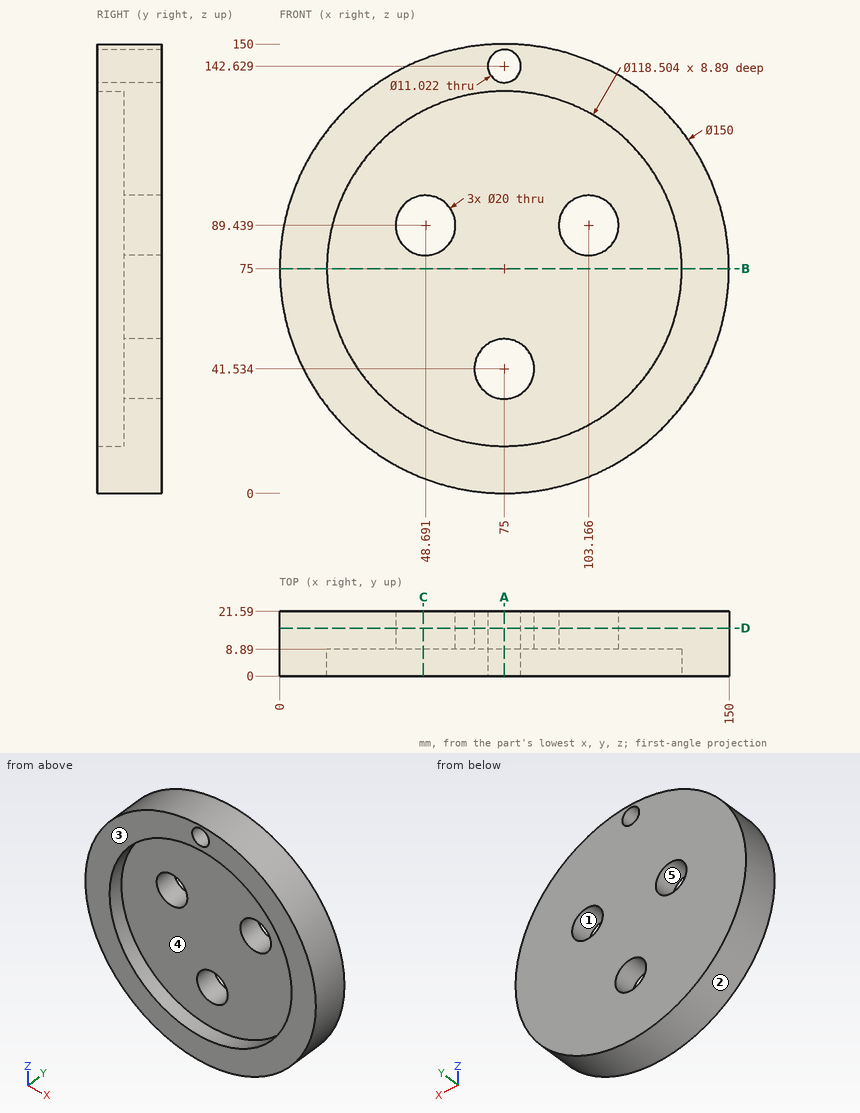
Can you work these out from the drawing? Everything is in mm from the part's minimum corner. A direction names the side the tool comes from. Round coordinates to 2 decimals unless told otherwise and drop trailing zeros. Write each loop counter-clockwise with the first axis right and the second up, starting at its lowest first coordinate (ties: lowest second). Pieces come first, ordered by that corner, then holes. Notation, with made-up numbers: (8.5, 45.5) - (63.5, 45.5) arc R20 cw to (63.5, 74.5) - close; hole circle Ø2 at (23.5, 62.25). An arc over 180 degrees is marked (long way). Put each result on its own line as item: value. Start each with the question number.
(1) Thinking about a two-plate mould opening in X: for the marked faces 1, 2 and 3, which applies, released by +X, released by -X, zero draft, split by the parting line, or undercut?
(2) I want a section at A-A, the plane x = 75. Please give me the cut outline in (y, z), plus the area to 3 significant figures.
(3) For the marked faces 4 and 5, which set-ups out of +Z, -Z, +X, -X, +Y, -Y let a thin tool reach every point of the face, with its end or its side?
(4) Will these pins go through, and if not, where does the flat tip stop? pin 1 (1 mm diameter, centred on x = 59, y = 17.5, fed in from +Z); pin 2 (1 mm diameter, centred on y = 18, z = 98.5, fed in from -X); pin 3 (3 mm diameter, centred on x = 57, z = 67.5, fed in from -Y); pin 4 (23 mm diameter, centred on x = 48.69, z = 89.44, fed in from +Y).
(5) I want a section at C-C, the plane x = 48. Please give me the cut outline in (y, z) (1 decimal).
(6) I need wall thicknesses on probe 1 along Z at (x, y) = (75, 2.5); probe 2 along Z at (x, y) = (77, 20.5) (1 decimal); probe 3 along Y at (x, z) = (102, 57). Which ranges of each line are inside material? Lowest first, please.
(7) I want a section at B-B, the plane z = 75. Please give me the cut outline in (x, y), plus the area to 4 significant figures.
(8) I want a section at D-D, the plane y = 16. Please give me the cut outline in (x, z).
Here are the results:
1. face 1: undercut
1. face 2: split by the parting line
1. face 3: zero draft
2. outline: (0, 0) - (21.59, 0) - (21.59, 31.53) - (8.89, 31.53) - (8.89, 15.75) - (0, 15.75) - close; (0, 134.25) - (8.89, 134.25) - (8.89, 51.53) - (21.59, 51.53) - (21.59, 137.12) - (0, 137.12) - close; (0, 148.14) - (21.59, 148.14) - (21.59, 150) - (0, 150) - close
2. area: 1,690 mm^2
3. face 4: -Y
3. face 5: +Y, -Y
4. pin 1: stops at z = 148.38
4. pin 2: stops at x = 3.61
4. pin 3: stops at y = 8.89
4. pin 4: stops at y = 21.59
5. outline: (0, 5) - (21.6, 5) - (21.6, 79.5) - (8.9, 79.5) - (8.9, 22.3) - (0, 22.3) - close; (0, 127.7) - (8.9, 127.7) - (8.9, 99.4) - (21.6, 99.4) - (21.6, 145) - (0, 145) - close
6. probe 1: z = 0 to 15.75, 134.25 to 137.12, 148.14 to 150
6. probe 2: z = 0 to 31.7, 51.3 to 137.5, 147.8 to 150
6. probe 3: y = 8.89 to 21.59
7. outline: (0, 0) - (15.75, 0) - (15.75, 8.89) - (134.25, 8.89) - (134.25, 0) - (150, 0) - (150, 21.59) - (0, 21.59) - close
7. area: 2,185 mm^2
8. outline: circle Ø150 at (75, 75); hole circle Ø20 at (48.69, 89.44); hole circle Ø20 at (75, 41.53); hole circle Ø11.02 at (75, 142.63); hole circle Ø20 at (103.17, 89.44)
